```python
from build123d import *

# Parameters (mm, degrees)
SKETCH_1_W               = 50
SKETCH_1_H               = 50
EXTRUDE_1_DEPTH          = 10
EXTRUDE_2_DEPTH          = 2.5
CUT_EXTRUDE_1_DEPTH      = 80.315824398
CUT_EXTRUDE_1_DEPTH_BACK = 80.315824398
SKETCH_5_R               = 1.75
CUT_EXTRUDE_3_DEPTH      = 80.315824398
CUT_EXTRUDE_3_DEPTH_BACK = 5
SKETCH_6_R               = 3.3
FILLET_1_R               = 10
SKETCH_8_R               = 5.5
CUT_EXTRUDE_5_DEPTH      = 6.5


with BuildPart() as part:
    # ｽｹｯﾁ1 → ﾎﾞｽ - 押し出し1 (new body)
    with BuildSketch(Plane(origin=(0, 0, 0), x_dir=(1, 0, 0), z_dir=(0, 1, 0))):
        Rectangle(SKETCH_1_W, SKETCH_1_H)
    extrude(amount=EXTRUDE_1_DEPTH)

    # ｽｹｯﾁ2 → ﾎﾞｽ - 押し出し2 (add, symmetric)
    with BuildSketch(Plane.XY):
        with BuildLine():
            Line((25, 46), (25, 10))
            Line((25, 10), (-25, 10))
            Line((-25, 10), (-25, 46))
            ThreePointArc((-25, 46), (0, 71), (25, 46))
        make_face()
    extrude(amount=EXTRUDE_2_DEPTH, both=True)

    # ｽｹｯﾁ5 → ｶｯﾄ - 押し出し1 (cut, two sides: drawn at the far end of the back side and taken through both)
    with BuildSketch(Plane.XY.offset(-CUT_EXTRUDE_1_DEPTH_BACK)):
        with Locations((0, 67)):
            Circle(SKETCH_5_R)
        with Locations((5.435199947, 66.284442352)):
            Circle(SKETCH_5_R)
        with Locations((10.5, 64.186533479)):
            Circle(SKETCH_5_R)
        with Locations((14.849242405, 60.849242405)):
            Circle(SKETCH_5_R)
        with Locations((18.186533479, 56.5)):
            Circle(SKETCH_5_R)
        with Locations((-18.186533479, 56.5)):
            Circle(SKETCH_5_R)
        with Locations((-14.849242405, 60.849242405)):
            Circle(SKETCH_5_R)
        with Locations((-10.5, 64.186533479)):
            Circle(SKETCH_5_R)
        with Locations((-5.435199947, 66.284442352)):
            Circle(SKETCH_5_R)
    extrude(amount=CUT_EXTRUDE_1_DEPTH + CUT_EXTRUDE_1_DEPTH_BACK, mode=Mode.SUBTRACT)

    # ｽｹｯﾁ6 → ｶｯﾄ - 押し出し3 (cut, two sides: drawn at the far end of the back side and taken through both)
    with BuildSketch(Plane(origin=(0, 0, 0), x_dir=(1, 0, 0), z_dir=(0, 1, 0)).offset(-CUT_EXTRUDE_3_DEPTH_BACK)):
        with Locations(Location((-10, -10, 0), (0, 0, 90))):
            Circle(SKETCH_6_R)
        with Locations(Location((10, -10, 0), (0, 0, 90))):
            Circle(SKETCH_6_R)
        with Locations(Location((10, 10, 0), (0, 0, 90))):
            Circle(SKETCH_6_R)
        with Locations(Location((-10, 10, 0), (0, 0, 90))):
            Circle(SKETCH_6_R)
    extrude(amount=CUT_EXTRUDE_3_DEPTH + CUT_EXTRUDE_3_DEPTH_BACK, mode=Mode.SUBTRACT)

    # ﾌｨﾚｯﾄ1
    fillet_1_edges = [part.edges().sort_by_distance(p)[0] for p in [
        (-25, 5, 25),
        (-25, 5, -25),
        (25, 5, -25),
        (25, 5, 25),
    ]]
    fillet(fillet_1_edges, radius=FILLET_1_R)

    # ｽｹｯﾁ8 → ｶｯﾄ - 押し出し5 (cut)
    with BuildSketch(Plane(origin=(0, 10, 0), x_dir=(1, 0, 0), z_dir=(0, 1, 0))):
        with Locations(Location((-10, -10, 0), (0, 0, 270))):
            Circle(SKETCH_8_R)
        with Locations(Location((10, -10, 0), (0, 0, 270))):
            Circle(SKETCH_8_R)
        with Locations(Location((10, 10, 0), (0, 0, 270))):
            Circle(SKETCH_8_R)
        with Locations(Location((-10, 10, 0), (0, 0, 270))):
            Circle(SKETCH_8_R)
    extrude(amount=-CUT_EXTRUDE_5_DEPTH, mode=Mode.SUBTRACT)


solid = part.part
```
CAD build for the part. Positions are in the model's coordinates, mm. A direction names the side the tool comes from. Coordinates: 2 decimals unless noted, no trailing zeros. Write each loop counter-clockwise with the first axis right and the second up, starting at its lowest first coordinate (ties: lowest second). Pieces come first, ordered by that corner, then holes. Notation, with made-up numbers: (-20.5, 8.25) -> (-0.5, 8.25) arc R19 cw to (-0.5, 31.25) -> close; hole circle Ø5 at (12.25, 17.5). An arc over 180 degrees is marked (long way). Return JSON: item names as keys, results as strings. Group by question number.
Q1. Which spindle directions (+Z, -Z, +X, -X, +Y, -Y) get a long thin tool onto all of the face, cutting with end or side? Do faces 5 (the face through (16.798, 55.435, -0.035)), 6 (the face through (-7.992, 1.726, -7.381)), 7 (the face through (7.89, 6.8, 15.08)), 8 (the face through (0, 41, -2.5)), 9 (the face through (0, 41, 2.5)). Say none if no direction does.
Q2. Cut at B-B, the plane z = 10. Give the cut face in (x, y).
Q3. Cut at C-C, the plane x = 10. Give the cut face in (y, z), then the cut area to 3 significant figures.
Q4. Drill centre lines: line 1 (X direction, y = 2.2, z = -10); line 2 (X direction, y = 8.75, z = 10); line 3 (Y direction, x = -21.5, z = -21). Where is each one in solid material? Low to high.
Q5. Cut at D-D, the plane y = 56.5. Give the cut face in (x, z), then the cut area to 3 significant figures.
Q6. Cut at A-A, the plane x = 0. Give the cut face in (y, z).
Q7. Pull direction Y, two halves, no side cores. Call faces 1 (the face through (10, 3.5, 14)), 2 (the face through (-12.11, 6.8, 15.08)), 3 (the face through (10.12, 62.48, -0.03)), 4 (the face through (14.47, 59.14, -0.03)): released by +Y, released by -Y, zero draft, split by the parting line, or undercut.
Q8. Flat gauge pins, fed straight in: pin 1 (12.5 mm diameter, centred on x = 10, z = -10, fed in from +Y); pin 2 (3 mm diameter, centred on x = -11, y = 47.5, fed in from -Z); pin 3 (1.5 mm diameter, centred on x = -10, z = -13, fed in from +Y). Where does each tip first touch, or does it go through?
Returned:
{
 "1": {"face 5": "+Z, -Z", "face 6": "+Y, -Y", "face 7": "+Y", "face 8": "-Z, +X, -X, +Y", "face 9": "+Z, +X, -X, +Y"},
 "2": {"outline": "(-25, 0) -> (-13.3, 0) -> (-13.3, 3.5) -> (-15.5, 3.5) -> (-15.5, 10) -> (-25, 10) -> close; (-6.7, 0) -> (6.7, 0) -> (6.7, 3.5) -> (4.5, 3.5) -> (4.5, 10) -> (-4.5, 10) -> (-4.5, 3.5) -> (-6.7, 3.5) -> close; (13.3, 0) -> (25, 0) -> (25, 10) -> (15.5, 10) -> (15.5, 3.5) -> (13.3, 3.5) -> close"},
 "3": {"outline": "(0, -25) -> (10, -25) -> (10, -15.5) -> (3.5, -15.5) -> (3.5, -13.3) -> (0, -13.3) -> close; (0, -6.7) -> (3.5, -6.7) -> (3.5, -4.5) -> (10, -4.5) -> (10, -2.5) -> (62.51, -2.5) -> (62.51, 2.5) -> (10, 2.5) -> (10, 4.5) -> (3.5, 4.5) -> (3.5, 6.7) -> (0, 6.7) -> close; (0, 13.3) -> (3.5, 13.3) -> (3.5, 15.5) -> (10, 15.5) -> (10, 25) -> (0, 25) -> close; (65.86, -2.5) -> (68.91, -2.5) -> (68.91, 2.5) -> (65.86, 2.5) -> close", "area": "589 mm2"},
 "4": {"line 1": "x = -25 to -13.3, -6.7 to 6.7, 13.3 to 25", "line 2": "x = -25 to -15.5, -4.5 to 4.5, 15.5 to 25", "line 3": "y = 0 to 10"},
 "5": {"outline": "(-22.69, -2.5) -> (-19.94, -2.5) -> (-19.94, 2.5) -> (-22.69, 2.5) -> close; (-16.44, -2.5) -> (16.44, -2.5) -> (16.44, 2.5) -> (-16.44, 2.5) -> close; (19.94, -2.5) -> (22.69, -2.5) -> (22.69, 2.5) -> (19.94, 2.5) -> close", "area": "192 mm2"},
 "6": {"outline": "(0, -25) -> (10, -25) -> (10, -2.5) -> (65.25, -2.5) -> (65.25, 2.5) -> (10, 2.5) -> (10, 25) -> (0, 25) -> close; (68.75, -2.5) -> (71, -2.5) -> (71, 2.5) -> (68.75, 2.5) -> close"},
 "7": {"face 1": "released by +Y", "face 2": "zero draft", "face 3": "undercut", "face 4": "undercut"},
 "8": {"pin 1": "stops at y = 10", "pin 2": "stops at z = -2.5", "pin 3": "stops at y = 3.5"}
}
